For this review, take the finished solid that the model builds, in its own axes (mm). Face numbers are marked on the shaded views. A direction names the side the tool comes from. Round coordinates to 2 decimals unless told otherwise and drop trailing zeros. Order: outer loops, then holes, each group sorted by start corner. A loop starts at its lowest first (then second) coordinate and runs counter-clockwise, first axis right, second up. Notation, with made-up numbers: (49.5, 81) - (92.5, 81) arc R4 ccw to (92.5, 87) - close; hole circle Ø3 at (-11, 88). An arc over 180 degrees is marked (long way). One line per question, with ' | ' between items.
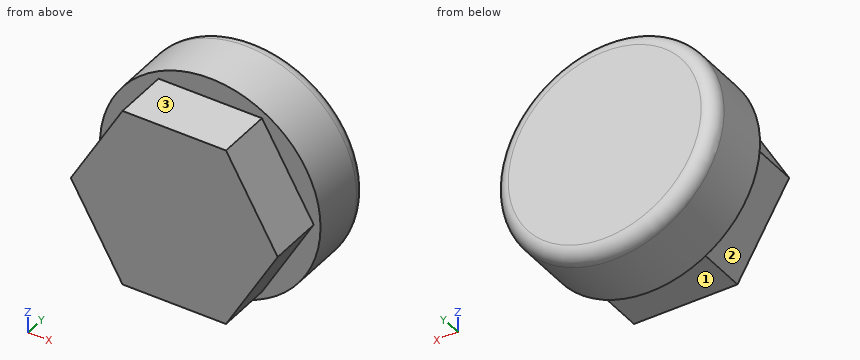
Autodesk Inventor part; units mm, degrees
ref_plane "YZ Plane" through (0, 0, 0) normal (1, 0, 0) x (0, 1, 0)
ref_plane "XZ Plane" through (0, 0, 0) normal (0, 1, 0) x (-1, 0, 0)
ref_plane "XY Plane" through (0, 0, 0) normal (0, 0, 1) x (1, 0, 0)
sketch "Sketch1" plane through (0, 0, 0) normal (0, 1, 0) x (-1, 0, 0)
  line L0 (3.7528, 0) -> (1.8764, -3.25)
  line L1 (1.8764, -3.25) -> (-1.8764, -3.25)
  line L2 (-1.8764, -3.25) -> (-3.7528, 0)
  line L3 (-3.7528, 0) -> (-1.8764, 3.25)
  line L4 (-1.8764, 3.25) -> (1.8764, 3.25)
  line L5 (1.8764, 3.25) -> (3.7528, 0)
  point P0 (0, 0)
  point P1 (0, 0)
  dimension "d0" = 6.5
extrude "Extrusion1" add sketch "Sketch1" along normal blind 2
sketch "Sketch2" plane through (0, 2, 0) normal (0, 1, 0) x (1, 0, 0)
  circle A0 centre (0, 0) radius 4
  dimension "d3" = 8
extrude "Extrusion2" add sketch "Sketch2" along normal blind 2.5
fillet "Fillet1" radius 0.5 1 edges at (-4, 4.5, 0)
properties part number "servo_nut_2_for_FatShark_180MG"
(1) We need section B-B on y = 0.85. State the section outline as (x, z) points, plus the area to 3 significant figures.
Output values:
outline: (-3.75, 0) - (-1.88, -3.25) - (1.88, -3.25) - (3.75, 0) - (1.88, 3.25) - (-1.88, 3.25) - close | area: 36.6 mm^2
(2) We need section C-C on y = 2.2. State the section outline as (x, z) points, plus the area to 3 significant figures.
Output values:
outline: circle Ø8 at (0, 0) | area: 50.3 mm^2
(3) Insertion check: pin 1 (1 mm diameter, centred on y = 3.5, z = -1.5, fed in from -X); pin 2 (0.6 mm diameter, centred on x = 0.5, y = 1, fed in from -Z); pin 3 (0.6 mm diameter, centred on x = 1, y = 1.5, fed in from +Z). Each pin has a flat end and moves straight along its axis. Give the tip position at first contact, or say it passes through.
Output values:
pin 1: x = -3.87 | pin 2: z = -3.25 | pin 3: z = 3.25
(4) For the marked faces 1, 2 and 3, list the 3-axis set-ups (+Z, -Z, +X, -X, +Y, -Y) from which the entire face can be reached by the end or side of a thin tool; tool diameter is ignored.
Output values:
face 1: -Z, +X, -X, -Y | face 2: -Z, -X, -Y | face 3: +Z, +X, -X, -Y
(5) For probe 1 along Z at (x, y) = (1.25, 4.2); probe 2 along Y at (x, z) = (2.75, 2); probe 3 along Z at (x, y) = (-2.25, 3.9), list the stretches that pass through material, from the lowest coordinate up. Write a range as [from, to].
Output values:
probe 1: [-3.76, 3.76] | probe 2: [2, 4.5] | probe 3: [-3.31, 3.31]
(6) We need section A-A on x = 0. State the section outline as (y, z) points.
Output values:
outline: (0, -3.25) - (2, -3.25) - (2, -4) - (4, -4) arc R0.5 ccw to (4.5, -3.5) - (4.5, 3.5) arc R0.5 ccw to (4, 4) - (2, 4) - (2, 3.25) - (0, 3.25) - close
